The listing builds one solid part. Answer for the finished solid, in the listing's coordinates (mm). Face numbers are marked on the shaded views. A direction names the side the tool comes from. Round coordinates to 2 decimals unless told otherwise and drop trailing zeros. Write each loop counter-clockwise with the first axis right and the second up, starting at its lowest first coordinate (ties: lowest second). Pieces come first, ordered by that corner, then holes.
(1) A cutting plane is placed at B-B, the plane x = -40.5. Give the vertices of the cut face in (y, z) (1 decimal), and give its area (3 significant figures).
(2) A cutting plane is placed at A-A, the plane z = 34.5. Give the vertices of the cut face in (x, y).
(3) Each of these flat-tipped pins is pushed along its axis until it touches: pin 1 Ø6 at (x, y) = (16, -12.5) entering from +Z; pin 2 Ø16 at (x, y) = (36.25, 0) entering from +Z; pin 3 Ø3 at (x, z) = (25.5, 25.5) entering from +Y. Where does it stop, or does it pass through?
(4) For the marked faces 1, 2 and 3, determine the directions among +Z, -Z, +X, -X, +Y, -Y from which every point of the face is accessible in a straight line to the end or side of a thin tool.
(5) A cutting plane is placed at D-D, the plane z = 4.5. Give the vertices of the cut face in (x, y).
(6) A cutting plane is placed at C-C, the plane x = -12. Give the vertices of the cut face in (y, z) (1 decimal).
(7) Find the intervals of material crossed by probe 1 along Z at (x, y) = (-46, 18); probe 2 along Y at (x, z) = (1.5, 21.5); probe 3 along X at (y, z) = (5.5, 4.5), in increasing order.
(8) The mould has two halves that part along X. Classify the marked faces 4, 5 and 6: +X half, -X half, draft (parallel to the pull), parting line (faces both ways), or undercut.
from build123d import *

# Parameters (mm, degrees)
CROQUIS1_R                = 10
SALIENTE_EXTRUIR1_DEPTH   = 7.9375
CROQUIS3_W                = 117.5
CROQUIS3_H                = 50
SALIENTE_EXTRUIR2_DEPTH   = 7.9375
CONVERTIR_S_LIDO1_START   = -58.75
CONVERTIR_S_LIDO1_DEPTH   = 117.5
CONVERTIR_S_LIDO1_2_DEPTH = 117.5


# Read off the part's stored shape, not the designer's step: Convertir-Sólido1
with BuildPart() as part:
    # Croquis1 → Saliente-Extruir1 (new body)
    with BuildSketch(Plane.XY):
        with BuildLine():
            ThreePointArc((58.75, 0), (52.159902577, 15.909902577), (36.25, 22.5))
            Line((36.25, 22.5), (-36.25, 22.5))
            ThreePointArc((-36.25, 22.5), (-52.159902577, 15.909902577), (-58.75, 0))
            Line((-58.75, 0), (-58.75, -47.992399286))
            Line((-58.75, -47.992399286), (58.75, -47.992399286))
            Line((58.75, -47.992399286), (58.75, 0))
        make_face()
        with Locations((-36.25, 0)):
            Circle(CROQUIS1_R, mode=Mode.SUBTRACT)
        with Locations((36.25, 0)):
            Circle(CROQUIS1_R, mode=Mode.SUBTRACT)
    extrude(amount=SALIENTE_EXTRUIR1_DEPTH)

    # Croquis3 → Saliente-Extruir2 (add)
    with BuildSketch(Plane.XZ.offset(47.992399286)):
        with Locations((0, 25)):
            Rectangle(CROQUIS3_W, CROQUIS3_H)
        with BuildLine():
            Line((-33.847495585, 39.845079108), (-33.847495585, 18.753600712))
            ThreePointArc((-33.847495585, 18.753600712), (-38.88030023, 13.720796067), (-43.913104875, 18.753600712))
            Line((-43.913104875, 18.753600712), (-43.913104875, 39.845079108))
            ThreePointArc((-43.913104875, 39.845079108), (-38.88030023, 44.877883753), (-33.847495585, 39.845079108))
        make_face(mode=Mode.SUBTRACT)
        with BuildLine():
            Line((36.463745774, 39.845079108), (36.463745774, 18.753600712))
            ThreePointArc((36.463745774, 18.753600712), (31.282917463, 13.572772401), (26.102089152, 18.753600712))
            Line((26.102089152, 18.753600712), (26.102089152, 39.845079108))
            ThreePointArc((26.102089152, 39.845079108), (31.282917463, 45.025907419), (36.463745774, 39.845079108))
        make_face(mode=Mode.SUBTRACT)
    extrude(amount=SALIENTE_EXTRUIR2_DEPTH)

    # Convertir-Sólido1 outline → Convertir-Sólido1 (cut)
    with BuildSketch(Plane.YZ.offset(CONVERTIR_S_LIDO1_START)):
        with BuildLine():
            ThreePointArc((-42.992399286, 0), (-52.140593268, 3.789306019), (-55.929899286, 12.9375))
            Line((-55.929899286, 12.9375), (-55.929899286, 0))
            Line((-55.929899286, 0), (-42.992399286, 0))
        make_face()
    extrude(amount=CONVERTIR_S_LIDO1_DEPTH, mode=Mode.SUBTRACT)

    # Convertir-S_lido1 2 outline → Convertir-S_lido1 2 (add)
    with BuildSketch(Plane.YZ.offset(CONVERTIR_S_LIDO1_START)):
        with BuildLine():
            ThreePointArc((-42.992399286, 7.9375), (-46.527933192, 9.401966094), (-47.992399286, 12.9375))
            Line((-47.992399286, 12.9375), (-47.992399286, 7.9375))
            Line((-47.992399286, 7.9375), (-42.992399286, 7.9375))
        make_face()
    extrude(amount=CONVERTIR_S_LIDO1_2_DEPTH)


solid = part.part
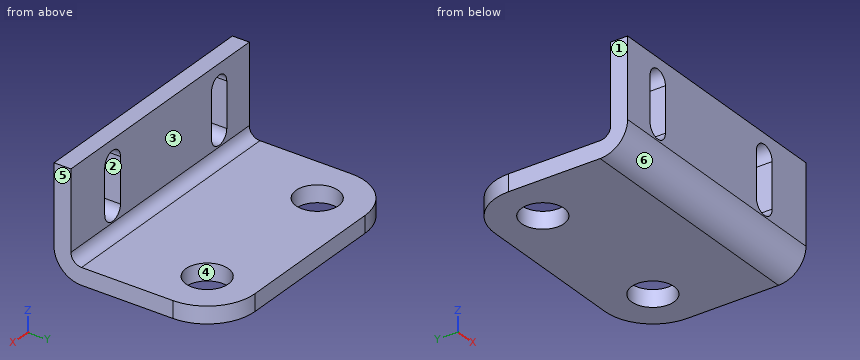
Solutions:
1. outline: (-55.9, 12.9) arc R12.9 ccw to (-43, 0) - (-9.1, 0) - (-9.1, 7.9) - (-43, 7.9) arc R5 cw to (-48, 12.9) - (-48, 14) - (-55.9, 14) - close; (-55.9, 44.6) - (-48, 44.6) - (-48, 50) - (-55.9, 50) - close; (9.1, 0) - (22.1, 0) - (22.1, 7.9) - (9.1, 7.9) - close
1. area: 536 mm2
2. outline: (-58.75, -55.93) - (-43.91, -55.93) - (-43.91, -47.99) - (-58.75, -47.99) - close; (-33.85, -55.93) - (26.1, -55.93) - (26.1, -47.99) - (-33.85, -47.99) - close; (36.46, -55.93) - (58.75, -55.93) - (58.75, -47.99) - (36.46, -47.99) - close
3. pin 1: stops at z = 7.94
3. pin 2: passes through
3. pin 3: stops at y = -47.99
4. face 1: +Z, -Z, -X, +Y, -Y
4. face 2: +Y, -Y
4. face 3: +Z, +X, -X, +Y
5. outline: (-58.75, -52.8) - (58.75, -52.8) - (58.75, 0) arc R22.5 ccw to (36.25, 22.5) - (-36.25, 22.5) arc R22.5 ccw to (-58.75, 0) - close; hole circle Ø20 at (-36.25, 0); hole circle Ø20 at (36.25, 0)
6. outline: (-55.9, 12.9) arc R12.9 ccw to (-43, 0) - (22.5, 0) - (22.5, 7.9) - (-43, 7.9) arc R5 cw to (-48, 12.9) - (-48, 50) - (-55.9, 50) - close
7. probe 1: z = 0 to 7.94
7. probe 2: y = -55.93 to -47.99
7. probe 3: x = -58.07 to -44.6, -27.9 to 27.9, 44.6 to 58.07
8. face 4: undercut
8. face 5: +X half
8. face 6: draft
